```python
from build123d import *

# Parameters (mm, degrees)
F0_W     = 87
F0_H     = 58
F1_DEPTH = 65
F2_W     = 10
F2_H     = 22
F3_DEPTH = 74
F4_W     = 9.5
F4_H     = 22
F4_W_2   = 30.5
F5_DEPTH = 58
F6_DEPTH = 90
F7_DEPTH = 99


with BuildPart() as f1:
    # F0 (on Top) → F1 (new body)
    with BuildSketch(Plane.XY):
        Rectangle(F0_W, F0_H)
    extrude(amount=F1_DEPTH)

    # F2 (on face) → F3 (cut)
    with BuildSketch(Plane(origin=(-43.5, 0, 0), x_dir=(0, -1, 0), z_dir=(-1, 0, 0))):
        with Locations((-7, 54)):
            Rectangle(F2_W, F2_H)
    extrude(amount=-F3_DEPTH, mode=Mode.SUBTRACT)

    # F4 (on face) → F5 (cut)
    with BuildSketch(Plane.XZ.offset(29)):
        with Locations((-4.75, 54)):
            Rectangle(F4_W, F4_H)
        with Locations((15.25, 54)):
            Rectangle(F4_W_2, F4_H)
    extrude(amount=-F5_DEPTH, mode=Mode.SUBTRACT)

    # F2 (on face) → F6 (cut)
    with BuildSketch(Plane(origin=(-43.5, 0, 0), x_dir=(0, -1, 0), z_dir=(-1, 0, 0))):
        with Locations((24, 54)):
            Rectangle(F2_W, F2_H)
    extrude(amount=-F6_DEPTH, mode=Mode.SUBTRACT)

    # F4 (on face) → F7 (cut)
    with BuildSketch(Plane.XZ.offset(29)):
        with BuildLine():
            ThreePointArc((1.5, 23), (1.0606601718, 24.0606601718), (0, 24.5))
            Line((0, 24.5), (0, 23))
            Line((0, 23), (1.5, 23))
        make_face()
        with BuildLine():
            ThreePointArc((0, 24.5), (-1.0606601718, 24.0606601718), (-1.5, 23))
            Line((-1.5, 23), (0, 23))
            Line((0, 23), (0, 24.5))
        make_face()
        with BuildLine():
            Line((0, 23), (-1.5, 23))
            ThreePointArc((-1.5, 23), (-1.0606601718, 21.9393398282), (0, 21.5))
            Line((0, 21.5), (0, 23))
        make_face()
        with BuildLine():
            Line((1.2536412571, 22.1763595454), (0, 23))
            Line((0, 23), (0, 21.5))
            ThreePointArc((0, 21.5), (0.7122286565, 21.6798748768), (1.2536412571, 22.1763595454))
        make_face()
        with BuildLine():
            Line((1.5, 23), (0, 23))
            Line((0, 23), (1.2536412571, 22.1763595454))
            ThreePointArc((1.2536412571, 22.1763595454), (1.4370911394, 22.5701522861), (1.5, 23))
        make_face()
    extrude(amount=-F7_DEPTH, mode=Mode.SUBTRACT)


solid = f1.part
```
Work out the finished part from the listing and answer in its coordinate system (mm). A direction names the side the tool comes from. Coordinates: 2 decimals unless noted, no trailing zeros. Write each loop counter-clockwise with the first axis right and the second up, starting at its lowest first coordinate (ties: lowest second). Pieces come first, ordered by that corner, then holes. Notation, with made-up numbers: (-18, 85.5) - (6, 85.5) arc R23 cw to (6, 106.5) - close; hole circle Ø8 at (-11, 38). An arc over 180 degrees is marked (long way). Answer as a JSON object with one key per item and string values.
Q1. Find section C-C (x = -20). Write down the section's boundary in (y, z).
Results list:
{"outline": "(-29, 0) - (29, 0) - (29, 65) - (12, 65) - (12, 43) - (2, 43) - (2, 65) - (-19, 65) - (-19, 43) - (-29, 43) - close"}
Q2. Which of the six approach directions +Z, -Z, +X, -X, +Y, -Y give full straight-line access (tool end or side, diameter ignored) to faces 1 (the flat face through (30.5, 5, 54)), 2 (the flat face through (-27, 12, 54)), 3 (the flat face through (-27, -19, 54))?
Results list:
{"face 1": "+Z, +Y, -Y", "face 2": "+Z, -X", "face 3": "+Z, +X, -X, -Y"}
Q3. Find section D-D (y = -6). Write down the section's boundary in (x, z), plus the area to 3 significant figures.
Results list:
{"outline": "(-43.5, 0) - (43.5, 0) - (43.5, 65) - (30.5, 65) - (30.5, 43) - (-9.5, 43) - (-9.5, 65) - (-43.5, 65) - close; hole circle Ø3 at (0, 23)", "area": "4,770 mm^2"}
Q4. Find section A-A (z = 49). Write down the section's boundary in (x, y).
Results list:
{"outline": "(-43.5, -19) - (-9.5, -19) - (-9.5, 2) - (-43.5, 2) - close; (-43.5, 12) - (-9.5, 12) - (-9.5, 29) - (-43.5, 29) - close; (30.5, -19) - (43.5, -19) - (43.5, 29) - (30.5, 29) - close"}
Q5. Given pin 1 Ø6.5 at (x, z) = (-35, 50) entering from -Y; pin 2 Ø4 at (x, y) = (13.5, 1.5) entering from +Z, each flat-ended and moving along its own axis, determine where each tip first touches the part or whether it passes through.
Results list:
{"pin 1": "stops at y = -19", "pin 2": "stops at z = 43"}
Q6. Find section B-B (y = 11). Write down the section's boundary in (x, z).
Results list:
{"outline": "(-43.5, 0) - (43.5, 0) - (43.5, 65) - (30.5, 65) - (30.5, 43) - (-43.5, 43) - close; hole circle Ø3 at (0, 23)"}
Q7. For a pull along X with two mould halves and no side action, classify faces 4 (the flat face through (-43.5, 0, 32)), 5 (the flat face through (-9.5, -9, 54)), 6 (the flat face through (43.5, 0, 32)), 7 (the flat face through (-27, 2, 54)) as pulls with the +X half, pulls with the -X half, needs draft (parallel to the pull), parting line crosses it, or undercut.
Results list:
{"face 4": "pulls with the -X half", "face 5": "undercut", "face 6": "pulls with the +X half", "face 7": "needs draft"}
Q8. Consider L1, parallel to X at y = -3, z = 46.5; L2, parallel to Y at x = -30.5, z = 55.5; L3, parallel to Z at x = 0.5, y = 5. Determine where each line is inside the solid, lowest interval first. Write a range as from..to.
Results list:
{"L1": "x = -43.5..-9.5, 30.5..43.5", "L2": "y = -19..2, 12..29", "L3": "z = 0..21.59, 24.41..43"}
